```python
from build123d import *

# Parameters (mm, degrees)
SKETCH1_R           = 12.5
BOSS_EXTRUDE1_DEPTH = 50
SKETCH2_R           = 1.75
BOSS_EXTRUDE2_DEPTH = 1


with BuildPart() as part:
    # Sketch1 → Boss-Extrude1 (new body)
    with BuildSketch(Plane(origin=(0, 0, 0), x_dir=(1, 0, 0), z_dir=(0, 1, 0))):
        with Locations(Location((0, 0, 0), (0, 0, 270))):
            Circle(SKETCH1_R)
    extrude(amount=BOSS_EXTRUDE1_DEPTH)

    # Sketch2 → Boss-Extrude2 (add)
    with BuildSketch(Plane(origin=(0, 50, 0), x_dir=(1, 0, 0), z_dir=(0, 1, 0))):
        with Locations(Location((0, 7.5, 0), (0, 0, 270))):
            Circle(SKETCH2_R)
        with Locations(Location((0, -7.5, 0), (0, 0, 270))):
            Circle(SKETCH2_R)
    extrude(amount=BOSS_EXTRUDE2_DEPTH)


solid = part.part
```
Verification items for the finished model (mm, model axes). A direction names the side the tool comes from. Give positions to 0.01 mm unless a question says otherwise; leave off trailing zeros. Loops run counter-clockwise (first coordinate to the right, second up) from the corner with the lowest first, then second, coordinate; pieces in that order, holes last.
1. Thickness scan on line 1 (Y direction, x = 8.75, z = -6.25); line 2 (Z direction, x = 0.5, y = 18.5); line 3 (Z direction, x = 2, y = 12.5). Record the ranges inside material, lowest first.
2. Set-up check for faces 1 (the cylindrical face through (0.526, 50.493, 9.169)), 2 (the flat face through (0, 51, -8)): record each of +Z, -Z, +X, -X, +Y, -Y from which the full face is reachable in a straight line by a thin tool's end or side.
3. Mould release check, pull along Z, two halves, no side actions. Record for faces 3 (the cylindrical face through (3.755, 24.65, 11.923)), 4 (the cylindrical face through (-0.67, 50.493, -5.883)), 5 (the flat face through (0, 0, 0)): released by +Z, released by -Z, zero draft, split by the parting line, or undercut.
4. Section check A-A, the plane z = 7.5. Enter the section's corners in (x, y), then the cut area to 3 significant figures.
5. Section check C-C, the plane y = 35.5. Enter the section's corners in (x, z), then the cut area to 3 significant figures.
6. Section check D-D, the plane z = 0. Enter the section's corners in (x, y).
7. Section check B-B, the plane x = 7.5. Enter the section's corners in (y, z).
8. Go/stop test with flat-tipped pins: pin 1 Ø1 at (x, y) = (4.5, 33.5) entering from +Z; pin 2 Ø12 at (x, y) = (7, 37.5) entering from -Z; pin 3 Ø3 at (x, y) = (-7, 28) entering from -Z (3 decimals). Record where each tip stops, or that it passes through.
Geometry says:
1. line 1: y = 0 to 50
1. line 2: z = -12.49 to 12.49
1. line 3: z = -12.34 to 12.34
2. face 1: +Y
2. face 2: +Z, -Z, +X, -X, +Y
3. face 3: split by the parting line
3. face 4: undercut
3. face 5: zero draft
4. outline: (-10, 0) - (10, 0) - (10, 50) - (1.75, 50) - (1.75, 51) - (-1.75, 51) - (-1.75, 50) - (-10, 50) - close
4. area: 1,000 mm2
5. outline: circle Ø25 at (0, 0)
5. area: 491 mm2
6. outline: (-12.5, 0) - (12.5, 0) - (12.5, 50) - (-12.5, 50) - close
7. outline: (0, -10) - (50, -10) - (50, 10) - (0, 10) - close
8. pin 1: stops at z = 11.84
8. pin 2: stops at z = -12.46
8. pin 3: stops at z = -11.225
